```python
from build123d import *

# Parameters (mm, degrees)
F1_DEPTH      = 7.112
F1_DEPTH_BACK = 7.112
F2_T1_DEPTH   = 38.654431888
F2_T3_DEPTH   = 71.8161099821
F2_T5_DEPTH   = 40.6320472649
F2_T7_DEPTH   = 71.8736907455
F2_T9_DEPTH   = 38.0679604185
F2_T11_DEPTH  = 41.2815855973


# Not quite as in the source:
# - a fillet or chamfer that OpenCascade refuses, or shapes differently, is made with other operations: its cross-section is extruded or revolved along the edge and cut away or added


with BuildPart() as f1:
    # F0 (on Front) → F1 (new body, two sides)
    with BuildSketch(Plane.XZ) as f1_sk:
        Polygon((0, 7.673737593), (-14.7832315415, 6.7385453665), (-14.7832315415, -5.9697437044), (0, -6.5452465788), align=None)
        Polygon((-14.7832315415, 6.7385453665), (-46.3809780777, 4.7396612354), (-46.3809780777, -4.7396612354), (-14.7832315415, -5.9697437044), align=None)
    extrude(amount=F1_DEPTH)
    extrude(f1_sk.sketch, amount=-F1_DEPTH_BACK)

    # F2: fillet of radius 5.08 on 8 edges, made by hand

    # F2_s2 → F2_t1 (cut)
    with BuildSketch(Plane.XZ.offset(-19.327215944)):
        with BuildLine():
            ThreePointArc((-46.3809780777, 0.1464251422), (-44.9622803199, -3.37511797), (-41.4985899316, -4.9297298549))
            Line((-41.4985899316, -4.9297298549), (-46.3809780777, -4.7396612354))
            Line((-46.3809780777, -4.7396612354), (-46.3809780777, 0.1464251422))
        make_face()
    extrude(amount=F2_T1_DEPTH, mode=Mode.SUBTRACT)

    # F2_s4 → F2_t3 (cut)
    with BuildSketch(Plane(origin=(-58.8169483786, 0, 2.2897106602), x_dir=(0, 1, 0), z_dir=(0.9992431097, 0, -0.0388999712))):
        with BuildLine():
            ThreePointArc((-7.112, -1.460292545), (-5.6241024484, -5.0523949934), (-2.032, -6.540292545))
            Line((-2.032, -6.540292545), (-7.112, -6.540292545))
            Line((-7.112, -6.540292545), (-7.112, -1.460292545))
        make_face()
        with BuildLine():
            ThreePointArc((7.112, -1.460292545), (5.6241024484, -5.0523949934), (2.032, -6.540292545))
            Line((2.032, -6.540292545), (7.112, -6.540292545))
            Line((7.112, -6.540292545), (7.112, -1.460292545))
        make_face()
    extrude(amount=F2_T3_DEPTH, mode=Mode.SUBTRACT)

    # F2_s6 → F2_t5 (cut)
    with BuildSketch(Plane.XZ.offset(-20.3160236325)):
        with BuildLine():
            ThreePointArc((0, -1.2636371258), (-1.5584568878, -4.924939368), (-5.2776118539, -6.3397921229))
            Line((-5.2776118539, -6.3397921229), (0, -6.5452465788))
            Line((0, -6.5452465788), (0, -1.2636371258))
        make_face()
    extrude(amount=F2_T5_DEPTH, mode=Mode.SUBTRACT)

    # F2_s8 → F2_t7 (cut)
    with BuildSketch(Plane(origin=(13.1581724385, 0, 0.8323904381), x_dir=(0, 1, 0), z_dir=(-0.9980050505, 0, -0.063134137))):
        with BuildLine():
            ThreePointArc((-2.032, -7.6584288737), (-5.6241024484, -6.1705313222), (-7.112, -2.5784288737))
            Line((-7.112, -2.5784288737), (-7.112, -7.6584288737))
            Line((-7.112, -7.6584288737), (-2.032, -7.6584288737))
        make_face()
        with BuildLine():
            ThreePointArc((7.112, -2.5784288737), (5.6241024484, -6.1705313222), (2.032, -7.6584288737))
            Line((2.032, -7.6584288737), (7.112, -7.6584288737))
            Line((7.112, -7.6584288737), (7.112, -2.5784288737))
        make_face()
    extrude(amount=F2_T7_DEPTH, mode=Mode.SUBTRACT)

    # F2_s10 → F2_t9 (cut)
    with BuildSketch(Plane.XZ.offset(-19.0339802092)):
        with BuildLine():
            ThreePointArc((-46.3809780777, -0.0291308483), (-45.0047373026, 3.4477308981), (-41.6216994935, 5.040734808))
            Line((-41.6216994935, 5.040734808), (-46.3809780777, 4.7396612354))
            Line((-46.3809780777, 4.7396612354), (-46.3809780777, -0.0291308483))
        make_face()
    extrude(amount=F2_T9_DEPTH, mode=Mode.SUBTRACT)

    # F2_s12 → F2_t11 (cut)
    with BuildSketch(Plane.XZ.offset(-20.6407927986)):
        with BuildLine():
            ThreePointArc((0, 2.2622204735), (-1.6031382536, 5.9659796985), (-5.4007214159, 7.3320861299))
            Line((-5.4007214159, 7.3320861299), (0, 7.673737593))
            Line((0, 7.673737593), (0, 2.2622204735))
        make_face()
    extrude(amount=F2_T11_DEPTH, mode=Mode.SUBTRACT)


solid = f1.part
```
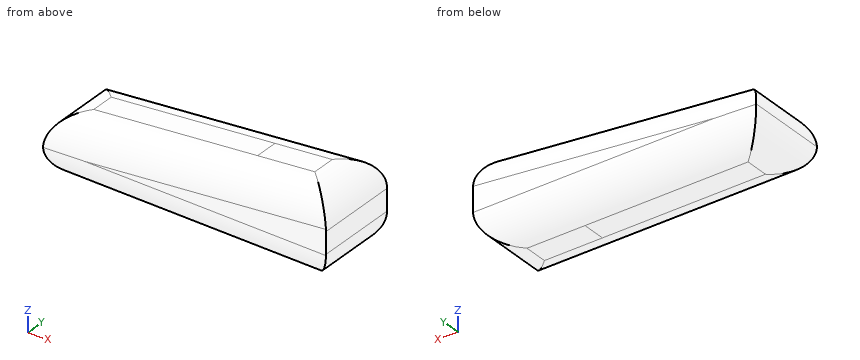
Input: part model. Units: mm. Frame: model coordinates. Round coordinates to 2 decimals unless told otherwise and drop trailing zeros. Order: outer loops, then holes, each group sorted by start corner. A loop starts at its lowest first (then second) coordinate and runs counter-clockwise, first axis right, second up. Notation, with made-up numbers: (40.25, -6) - (64.25, -6) arc R28 ccw to (64.25, 30) - close; hole circle Ø11 at (-38, -31.5). An arc over 180 degrees is marked (long way). One line per question, with ' | ' between items. Start each with the question number.
1) Cut plane B-B, the plane y = 3.5. Return the cut outline in (x, z), then the cut area to 3 significant figures.
2) Contact query for flat-ended pins moving along their axis: P1, Ø3, axis at x = -24, y = 4.5, coming from the -Z side; P2, Ø1.5, axis at x = -36.5, y = -0.5, coming from the +Z side; P3, Ø4, axis at x = -35, y = 3.5, coming from the -Z side. Output: stop coordinate, or through.
3) Cut plane A-A, the plane y = -1. Return the cut outline in (x, z), then the cut area to 3 significant figures.
4) Cut plane C-C, the plane y = -4.75. Return the cut outline in (x, z).
5) Ray query, probe 1 along Y at (x, z) = (-10.5, -1.25); probe 2 along X at (y, z) = (4.5, 0); probe 3 along X at (y, z) = (-0.25, 1.25). Return the intervals inside material, ascending.
Worked out:
1) outline: (-46.38, 0.06) arc R5.08 ccw to (-42.96, -4.66) - (-3.8, -6.18) arc R5.08 ccw to (0, -1.26) - (0, 2.26) arc R5.08 ccw to (-3.92, 7.21) - (-43.07, 4.73) arc R5.08 ccw to start | area: 511 mm^2
2) P1: stops at z = -5.52 | P2: stops at z = 5.41 | P3: stops at z = -5.24
3) outline: (-46.38, 0.06) arc R5.08 ccw to (-41.5, -4.93) - (-5.28, -6.34) arc R5.08 ccw to (0, -1.26) - (0, 2.26) arc R5.08 ccw to (-5.4, 7.33) - (-41.62, 5.04) arc R5.08 ccw to start | area: 527 mm^2
4) outline: (-46.38, 0.06) arc R5.08 ccw to (-44.18, -4.04) - (-2.53, -5.66) arc R5.08 ccw to (0, -1.26) - (0, 2.26) arc R5.08 ccw to (-2.64, 6.72) - (-44.28, 4.08) arc R5.08 ccw to start
5) probe 1: y = -7.11 to 7.11 | probe 2: x = -46.38 to 0 | probe 3: x = -46.22 to 0
